The model under review builds one solid part; all positions refer to its coordinate system, in mm. A direction names the side the tool comes from. Give positions to 0.01 mm unless a question says otherwise; leave off trailing zeros. Order: outer loops, then holes, each group sorted by start corner. A loop starts at its lowest first (then second) coordinate and runs counter-clockwise, first axis right, second up.
Autodesk Inventor part; units mm, degrees
ref_plane "YZ Plane" through (0, 0, 0) normal (1, 0, 0) x (0, 1, 0)
ref_plane "XZ Plane" through (0, 0, 0) normal (0, 1, 0) x (-1, 0, 0)
ref_plane "XY Plane" through (0, 0, 0) normal (0, 0, 1) x (1, 0, 0)
sketch "PanelDimension" plane through (0, 0, 0) normal (0, 0, 1) x (1, 0, 0)
  line L0 (-187.5, 125) -> (187.5, 125)
  line L1 (187.5, 125) -> (187.5, -125)
  line L2 (187.5, -125) -> (-187.5, -125)
  line L3 (-187.5, -125) -> (-187.5, 125)
  point P0 (0, 0)
  point P1 (-187.5, 0)
  point P2 (0, 125)
  dimension "d0" = 375
  dimension "d2" = 250
extrude "BodyExtrusion" add sketch "PanelDimension" along normal blind 75
sketch "PanelInside" plane through (0, 0, 75) normal (0, 0, 1) x (1, 0, 0)
  line L0 (187.5, 125) -> (-187.5, 125)
  line L1 (-187.5, 125) -> (-187.5, -125)
  line L2 (-162.5, 100) -> (162.5, 100)
  line L3 (162.5, 100) -> (162.5, -100)
  line L4 (162.5, -100) -> (-162.5, -100)
  line L5 (-162.5, -100) -> (-162.5, 100)
  point P0 (0, 0)
  point P1 (-162.5, 0)
  point P2 (0, 100)
  dimension "d7" = 25
  dimension "d8" = 25
extrude "CavityExtrusion" cut sketch "PanelInside" against normal blind 50
fillet "BodyOutsideFillet" radius 2 4 edges at (-187.5, 125, 37.5) (187.5, 125, 37.5) (187.5, -125, 37.5) (-187.5, -125, 37.5)
fillet "BodyInsideFillet" radius 2 4 edges at (162.5, 100, 50) (-162.5, 100, 50) (-162.5, -100, 50) (162.5, -100, 50)
properties part number "Panel_Body"
Item 1: For faces 1 (the flat face through (-2, 1, 25)), 2 (the flat face through (3, -125, 37)), list the 3-axis set-ups (+Z, -Z, +X, -X, +Y, -Y) from which the entire face can be reached by the end or side of a thin tool; tool diameter is ignored.
Values found:
face 1: +Z
face 2: +Z, -Z, +X, -X, -Y
Item 2: Take a section at A-A (z = 64.5). Give the boundary of the cut face in (x, y).
Values found:
outline: (-187.5, -123) arc R2 ccw to (-185.5, -125) - (185.5, -125) arc R2 ccw to (187.5, -123) - (187.5, 123) arc R2 ccw to (185.5, 125) - (-185.5, 125) arc R2 ccw to (-187.5, 123) - close; hole (-162.5, -98) arc R2 ccw to (-160.5, -100) - (160.5, -100) arc R2 ccw to (162.5, -98) - (162.5, 98) arc R2 ccw to (160.5, 100) - (-160.5, 100) arc R2 ccw to (-162.5, 98) - close
Item 3: Take a section at B-B (y = -20). Give the boundary of the cut face in (x, z).
Values found:
outline: (-187.5, 0) - (187.5, 0) - (187.5, 75) - (162.5, 75) - (162.5, 25) - (-162.5, 25) - (-162.5, 75) - (-187.5, 75) - close
Item 4: For line 1 (X direction, y = -49.5, z = 59); line 2 (Y direction, x = 85, z = 52.5); line 3 (Z direction, x = 135.5, y = -63), list the stretches that pass through material, from the lowest coordinate up.
Values found:
line 1: x = -187.5 to -162.5, 162.5 to 187.5
line 2: y = -125 to -100, 100 to 125
line 3: z = 0 to 25
Item 5: Draft analysis for pull direction X (two halves, no side actions). For faces 3 (the flat face through (-162.5, -1, 50)), 4 (the flat face through (-3, -109, 75)), 5 (the flat face through (-187.5, -2, 37)), 6 (the flat face through (162.5, 1, 50)), state which applies: released by +X, released by -X, zero draft, split by the parting line, or undercut.
Values found:
face 3: undercut
face 4: zero draft
face 5: released by -X
face 6: undercut
Item 6: Take a section at C-C (x = -84.5). Give the boundary of the cut face in (y, z).
Values found:
outline: (-125, 0) - (125, 0) - (125, 75) - (100, 75) - (100, 25) - (-100, 25) - (-100, 75) - (-125, 75) - close
Item 7: Clearance check with a flat-ended pin moving along its axis: pin 1 Ø5 at (x, y) = (-139.5, -66.5) entering from +Z. State where the tip first meets the part, or that it passes through.
Values found:
pin 1: stops at z = 25
